Can you work these out from the model? Positions are in its coordinate system, mm. Face numbers are marked on the shaded views. A direction names the side the tool comes from. Round coordinates to 2 decimals unless told otherwise and drop trailing zeros. Write each loop counter-clockwise with the first axis right and the second up, starting at its lowest first coordinate (ties: lowest second). Pieces come first, ordered by that corner, then holes. Notation, with made-up numbers: M 50,58.25 L 108,58.25 A28 ccw 108,89.25 Z; hole C 74,9 d8. An arc over 180 degrees is marked long. Answer as a JSON object with one key per item and string values. Group by question number.
1) Suppose I cut it at B-B, the plane y = -13.55. Write out the boundary of the cut face in (x, z), and give its area (3 significant figures).
2) Suppose I cut it at D-D, the plane z = 11.25. Write out the boundary of the cut face in (x, y), and give its area (3 significant figures).
3) If we mould it in two halves opening along X, with no side actions, what happens to the marked faces 5, 6 and 7? For each: +X half, -X half, draft (parallel to the pull), parting line (faces both ways), or undercut.
4) Suppose I cut it at A-A, the plane x = 13.75. Write out the boundary of the cut face in (y, z), and give its area (3 significant figures).
5) On a 3-axis mill with a long thin cutter (end or side, diameter ignored), from which of +Z, -Z, +X, -X, +Y, -Y can I reach the whole of each face in a straight line? I mean the marked faces 1, 2, 3 and 4. Say none if no direction works.
6) Please list where these lines run through material, in increasing order: L1, parallel to Y at x = 13.85, z = 8; L2, parallel to X at y = -10.25, z = 12.5; L3, parallel to Y at x = 5.25, z = 8. Write a range as [from, to].
7) Suppose I cut it at C-C, the plane z = 8. Write out the boundary of the cut face in (x, y), and give its area (3 significant figures).
8) I'm going to push flat-ended pins straight in: pin 1 Ø0.5 at (x, z) = (8, 0.5) entering from -Y; pin 2 Ø1.8 at (x, z) = (6, 14.5) entering from -Y. Where does each tip first touch, or does it pass through?
Autodesk Inventor part; units mm, degrees
ref_plane "Work Plane5" through (7.5, -3.5, 0) normal (0, -1, 0) x (1, 0, 0)
ref_plane "YZ Plane" through (0, 0, 0) normal (1, 0, 0) x (0, 1, 0)
ref_plane "XZ Plane" through (0, 0, 0) normal (0, 1, 0) x (-1, 0, 0)
sketch "Sketch1" plane through (0, 0, 0) normal (0, 0, 1) x (1, 0, 0)
  line L0 (0, 0) -> (15, 0)
  line L1 (15, 0) -> (15, -16)
  line L2 (15, -16) -> (0, -16)
  line L3 (0, -16) -> (0, 0)
  dimension "d0" = 16
  dimension "d1" = 15
extrude "Extrusion1" add sketch "Sketch1" along normal blind 16
sketch "Sketch21" plane through (0, 0, 0) normal (0, 0, -1) x (-1, 0, 0)
  circle A0 centre (-7.5, -8) radius 4.5
  line L0 (0, 0) -> (0, -16)
  line L1 (-15, 0) -> (0, 0)
  dimension "d2" = 16
  dimension "d89" = 9
  dimension "d90" = 7.5
  dimension "d91" = 8
extrude "Extrusion12" add sketch "Sketch21" along normal blind 10
sketch "Sketch22" plane through (7.5, -8, -10) normal (0, 0, -1) x (-1, 0, 0)
  ellipse E0 centre (0, 0) end of major axis (0, -3) minor radius 1.8
  point P0 (7.5, 8)
  dimension "d2" = 16
  dimension "d94" = 1.8
  dimension "d95" = 3
extrude "Extrusion13" cut sketch "Sketch22" against normal blind 8
ref_plane "Work Plane5" through (7.5, -3.5, 0) normal (0, -1, 0) x (1, 0, 0)
sketch "Sketch24" plane through (7.5, -3.5, 0) normal (0, -1, 0) x (1, 0, 0)
  line L0 (-4.5, -10) -> (4.5, -10)
  line L1 (4.5, -10) -> (-4.5, -10)
  line L2 (-4.5, -10) -> (-4.5, -7)
  line L3 (-4.5, 0) -> (-4.5, -10)
  line L4 (4.5, -10) -> (4.5, -7)
  line L5 (4.5, 0) -> (4.5, -10)
  arc A0 (-4.5, -7) -> (4.5, -7) centre (0, -0.3856) ccw
  point P0 (-7.5, 0)
  dimension "d2" = 16
  dimension "d98" = 3
  dimension "d99" = 3
  dimension "d100" = 8
extrude "Extrusion14" cut sketch "Sketch24" along normal blind 12
sketch "Sketch31" plane through (0, 0, 16) normal (0, 0, 1) x (1, 0, 0)
  line L0 (4.5, -3) -> (10.5, -3)
  line L1 (10.5, -3) -> (10.5, -6.1)
  line L2 (10.5, -6.1) -> (4.5, -6.1)
  line L3 (4.5, -6.1) -> (4.5, -3)
  line L4 (15, -16) -> (15, 0)
  line L5 (15, 0) -> (0, 0)
  dimension "d2" = 16
  dimension "d130" = 3.1
  dimension "d131" = 6
  dimension "d132" = 4.5
  dimension "d133" = 3
extrude "Extrusion20" cut sketch "Sketch31" against normal blind 6
sketch "Sketch32" plane through (0, 0, 16) normal (0, 0, 1) x (1, 0, 0)
  line L0 (4, -7.284) -> (11, -7.284)
  line L1 (11, -7.284) -> (11, -16.284)
  line L2 (11, -16.284) -> (4, -16.284)
  line L3 (4, -16.284) -> (4, -7.284)
  line L4 (10.5, -6.1) -> (4.5, -6.1)
  line L5 (15, -16) -> (15, 0)
  point P0 (0, 0)
  dimension "d2" = 16
  dimension "d140" = 7
  dimension "d141" = 1.184
  dimension "d142" = 4
  dimension "d143" = 9
extrude "Extrusion21" cut sketch "Sketch32" against normal blind 15
sketch "Sketch33" plane through (0, -16, 0) normal (-1, 0, 0) x (0, 0, 1)
  circle A0 centre (8, 11.45) radius 1.2
  line L0 (16, 0) -> (16, 16)
  point P0 (0, 16)
  dimension "d2" = 16
  dimension "d146" = 2.4
  dimension "d147" = 8
  dimension "d148" = 4.55
extrude "Extrusion22" cut sketch "Sketch33" against normal through all
sketch "Sketch34" plane through (0, 0, 0) normal (0, 0, -1) x (-1, 0, 0)
  line L0 (0, -16) -> (-15, -16)
  line L1 (-11, -16) -> (-4, -16)
  line L2 (-4, -16) -> (-4, -12.9958)
  line L3 (-4, -12.9958) -> (-11, -12.9958)
  line L4 (-11, -12.9958) -> (-11, -16)
  line L5 (0, 0) -> (0, -16)
  dimension "d2" = 16
  dimension "d151" = 7
  dimension "d152" = 4
extrude "Extrusion23" cut sketch "Sketch34" against normal blind 10
sketch "Sketch35" plane through (15, -16, 0) normal (1, 0, 0) x (0, 0, -1)
  circle A0 centre (-8, 2.45) radius 1.2
  line L0 (0, 0) -> (-16, 0)
  line L1 (-16, 0) -> (-16, 16)
  point P0 (0, 16)
  dimension "d2" = 16
  dimension "d155" = 2.4
  dimension "d156" = 2.45
  dimension "d157" = 8
extrude "Extrusion24" cut sketch "Sketch35" against normal through all
fillet "Fillet4" radius 3 1 edges at (7.5, 0, 0)
properties part number "korob_3" material "ABS Plastic"
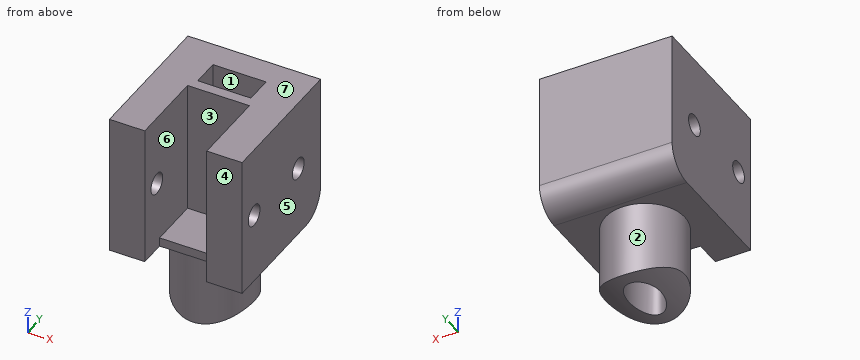
Results:
{
 "1": {"outline": "M 0,0 L 4,0 L 4,6.8 L 0,6.8 Z; M 0,9.2 L 4,9.2 L 4,16 L 0,16 Z; M 11,0 L 15,0 L 15,6.8 L 11,6.8 Z; M 11,9.2 L 15,9.2 L 15,16 L 11,16 Z", "area": "109 mm^2"},
 "2": {"outline": "M 0,-16 L 4,-16 L 4,-7.28 L 11,-7.28 L 11,-16 L 15,-16 L 15,0 L 0,0 Z; hole M 4.5,-6.1 L 10.5,-6.1 L 10.5,-3 L 4.5,-3 Z", "area": "160 mm^2"},
 "3": {"face 5": "+X half", "face 6": "undercut", "face 7": "draft"},
 "4": {"outline": "M -16,0 L -3,0 A3 ccw 0,3 L 0,16 L -16,16 Z; hole C -13.55,8 d2.4; hole C -4.55,8 d2.4", "area": "245 mm^2"},
 "5": {"face 1": "+Z", "face 2": "-Z", "face 3": "+Z, -Y", "face 4": "+Z, -Z, +X, -X, -Y"},
 "6": {"L1": "[-16, -14.75], [-12.35, -5.75], [-3.35, 0]", "L2": "[0, 4], [11, 15]", "L3": "[-7.28, -5.75], [-3.35, 0]"},
 "7": {"outline": "M 0,-16 L 4,-16 L 4,-14.75 L 0,-14.75 Z; M 0,-12.35 L 4,-12.35 L 4,-7.28 L 11,-7.28 L 11,-12.35 L 15,-12.35 L 15,-5.75 L 0,-5.75 Z; M 0,-3.35 L 15,-3.35 L 15,0 L 0,0 Z; M 11,-16 L 15,-16 L 15,-14.75 L 11,-14.75 Z", "area": "124 mm^2"},
 "8": {"pin 1": "y = -13", "pin 2": "y = -7.28"}
}
